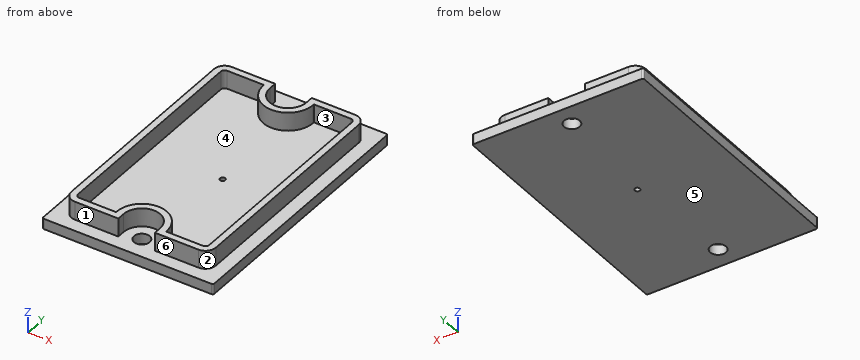
Autodesk Inventor part; units mm, degrees
ref_plane "YZ Plane" through (0, 0, 0) normal (1, 0, 0) x (0, 1, 0)
ref_plane "XZ Plane" through (0, 0, 0) normal (0, 1, 0) x (-1, 0, 0)
ref_plane "XY Plane" through (0, 0, 0) normal (0, 0, 1) x (1, 0, 0)
sketch "Sketch1" plane through (0, 0, 0) normal (0, 0, 1) x (1, 0, 0)
  circle A0 centre (-1.4563, -20.8) radius 1.5
  circle A1 centre (-1.4563, 20.8) radius 1.5
  line L0 (14.8852, 24.5) -> (14.8852, -24.5)
  arc A2 (14.8852, 24.5) -> (14.5437, 24.8416) centre (14.5437, 24.5) ccw
  line L1 (-17.4563, 24.8416) -> (14.5437, 24.8416)
  arc A3 (-17.4563, 24.8416) -> (-17.7979, 24.5) centre (-17.4563, 24.5) ccw
  line L2 (-17.7979, -24.5) -> (-17.7979, 24.5)
  arc A4 (-17.7979, -24.5) -> (-17.4563, -24.8416) centre (-17.4563, -24.5) ccw
  line L3 (14.5437, -24.8416) -> (-17.4563, -24.8416)
  arc A5 (14.5437, -24.8416) -> (14.8852, -24.5) centre (14.5437, -24.5) ccw
  line L4 (-13.2563, 22.3) -> (-4.9563, 22.3)
  line L5 (-4.9563, 22.3) -> (-4.9563, 20.8)
  arc A6 (-4.9563, 20.8) -> (2.0437, 20.8) centre (-1.4563, 20.8) ccw
  line L6 (2.0437, 20.8) -> (2.0437, 22.3)
  line L7 (2.0437, 22.3) -> (10.3437, 22.3)
  arc A7 (12.3437, 20.3) -> (10.3437, 22.3) centre (10.3437, 20.3) ccw
  line L8 (12.3437, 20.3) -> (12.3437, -20.3)
  arc A8 (10.3437, -22.3) -> (12.3437, -20.3) centre (10.3437, -20.3) ccw
  line L9 (10.3437, -22.3) -> (2.0437, -22.3)
  line L10 (2.0437, -22.3) -> (2.0437, -20.8)
  arc A9 (2.0437, -20.8) -> (-4.9563, -20.8) centre (-1.4563, -20.8) ccw
  line L11 (-4.9563, -20.8) -> (-4.9563, -22.3)
  line L12 (-4.9563, -22.3) -> (-13.2563, -22.3)
  arc A10 (-15.2563, -20.3) -> (-13.2563, -22.3) centre (-13.2563, -20.3) ccw
  line L13 (-15.2563, -20.3) -> (-15.2563, 20.3)
  arc A11 (-13.2563, 22.3) -> (-15.2563, 20.3) centre (-13.2563, 20.3) ccw
  circle A12 centre (-1.4563, 20.8) radius 1.5
  circle A13 centre (-1.4563, -20.8) radius 1.5
  arc A14 (-17.4563, 26.5) -> (-19.4563, 24.5) centre (-17.4563, 24.5) ccw
  line L14 (-19.4563, -24.5) -> (-19.4563, 24.5)
  arc A15 (-19.4563, -24.5) -> (-17.4563, -26.5) centre (-17.4563, -24.5) ccw
  line L15 (14.5437, -26.5) -> (-17.4563, -26.5)
  arc A16 (14.5437, -26.5) -> (16.5437, -24.5) centre (14.5437, -24.5) ccw
  line L16 (16.5437, 24.5) -> (16.5437, -24.5)
  arc A17 (16.5437, 24.5) -> (14.5437, 26.5) centre (14.5437, 24.5) ccw
  line L17 (-17.4563, 26.5) -> (14.5437, 26.5)
  arc A18 (-6.2217, 20.8) -> (3.3091, 20.8) centre (-1.4563, 20.8) ccw
  line L18 (-6.2217, 20.8) -> (-6.2217, 21.0346)
  line L19 (-6.2217, 21.0346) -> (-13.2563, 21.0346)
  arc A19 (-13.2563, 21.0346) -> (-13.9909, 20.3) centre (-13.2563, 20.3) ccw
  line L20 (-13.9909, 20.3) -> (-13.9909, -20.3)
  arc A20 (-13.9909, -20.3) -> (-13.2563, -21.0346) centre (-13.2563, -20.3) ccw
  line L21 (-13.2563, -21.0346) -> (-6.2217, -21.0346)
  line L22 (-6.2217, -21.0346) -> (-6.2217, -20.8)
  arc A21 (3.3091, -20.8) -> (-6.2217, -20.8) centre (-1.4563, -20.8) ccw
  line L23 (3.3091, -20.8) -> (3.3091, -21.0346)
  line L24 (3.3091, -21.0346) -> (10.3437, -21.0346)
  arc A22 (10.3437, -21.0346) -> (11.0783, -20.3) centre (10.3437, -20.3) ccw
  line L25 (11.0783, -20.3) -> (11.0783, 20.3)
  arc A23 (11.0783, 20.3) -> (10.3437, 21.0346) centre (10.3437, 20.3) ccw
  line L26 (10.3437, 21.0346) -> (3.3091, 21.0346)
  line L27 (3.3091, 21.0346) -> (3.3091, 20.8)
  point P0 (0, 0)
  point P1 (0, 0)
  point P2 (0, 0)
extrude "Extrusion1" add sketch "Sketch1" along normal blind 2 contours L0 A5 L3 A4 L2 A3 L1 A2
extrude "Extrusion2" add sketch "Sketch1" along normal blind 5.5 contours L4 L5 A6 L6 L7 A7 L8 A8 L9 L10 A9 L11 L12 A10 L13 A11
extrude "Extrusion3" add sketch "Sketch1" along normal blind 2 contours A18 L27 L26 A23 L25 A22 L24 L23 A21 L22 L21 A20 L20 A19 L19 L18
sketch "Sketch2" plane through (0, 0, 2) normal (0, 0, 1) x (1, 0, 0)
  circle A0 centre (0, 0) radius 0.5
  dimension "d6" = 1
extrude "Extrusion4" cut sketch "Sketch2" along normal through all both and the other way through all
properties part number "Goma"
Source: CAD feature listing. Evaluate the final solid. Frame: model axes, mm. Face numbers are marked on the shaded views. A direction names the side the tool comes from. Give positions to 0.01 mm unless a question says otherwise; leave off trailing zeros. Order: outer loops, then holes, each group sorted by start corner. A loop starts at its lowest first (then second) coordinate and runs counter-clockwise, first axis right, second up. Notation, with made-up numbers: (41.5, -10.75) -> (85.5, -10.75) arc R9 ccw to (85.5, -1.75) -> close; hole circle Ø1 at (61.25, 80). An arc over 180 degrees is marked (long way). Write item = value, one per line.
Item 1: Ray query, probe 1 along X at (y, z) = (-11, 3.55); probe 2 along Y at (x, z) = (-3.5, 3.05); probe 3 along Z at (x, y) = (9, -14). Return the intervals inside material, ascending.
Check result:
probe_1 = -15.26 to -13.99, 11.08 to 12.34
probe_2 = -17.96 to -16.5, 16.5 to 17.96
probe_3 = 0 to 2
Item 2: Section query B-B (y = 0). Output: boundary loops of the cut face in (x, z).
Check result:
outline = (-17.8, 0) -> (-0.5, 0) -> (-0.5, 2) -> (-13.99, 2) -> (-13.99, 5.5) -> (-15.26, 5.5) -> (-15.26, 2) -> (-17.8, 2) -> close; (0.5, 0) -> (14.89, 0) -> (14.89, 2) -> (12.34, 2) -> (12.34, 5.5) -> (11.08, 5.5) -> (11.08, 2) -> (0.5, 2) -> close
Item 3: Section query C-C (y = -10). Output: boundary loops of the cut face in (x, z).
Check result:
outline = (-17.8, 0) -> (14.89, 0) -> (14.89, 2) -> (12.34, 2) -> (12.34, 5.5) -> (11.08, 5.5) -> (11.08, 2) -> (-13.99, 2) -> (-13.99, 5.5) -> (-15.26, 5.5) -> (-15.26, 2) -> (-17.8, 2) -> close
Item 4: Set-up query: the marked faces 1, 2 and 3. Return all of +Z, -Z, +X, -X, +Y, -Y with unobstructed straight access to the full face (end or side cutting, diameter ignored); none if empty.
Check result:
face_1 = +Z, +X, -X, -Y
face_2 = +Z, +X, -Y
face_3 = +Z
Item 5: Contact query for flat-ended pins moving along their axis: pin 1 (1 mm diameter, centred on y = -5.5, z = 3, fed in from +X); pin 2 (7.5 mm diameter, centred on x = -1, y = 0, fed in from +Z); pin 3 (0.8 mm diameter, centred on y = -21.5, z = 3, fed in from +X). Output: stop coordinate, or through.
Check result:
pin_1 = 12.34
pin_2 = 2
pin_3 = 12.18
Item 6: Mould query, pull axis Y, two halves, no side actions, for the marked faces 4, 5 and 6. Classes: +Y half, -Y half, draft (parallel to the pull), parting line (faces both ways), or undercut.
Check result:
face_4 = undercut
face_5 = draft
face_6 = -Y half
